Build history of the part. All positions in model axes, mm. A direction names the side the tool comes from. Round coordinates to 2 decimals unless told otherwise and drop trailing zeros. Write each loop counter-clockwise with the first axis right and the second up, starting at its lowest first coordinate (ties: lowest second). Pieces come first, ordered by that corner, then holes.
1) Saw through at A-A (z = 0). Write the cut outline in (x, y).
2) Which spindle directions (+Z, -Z, +X, -X, +Y, -Y) get a long thin tool onto all of the face, cutting with end or side? Do faces 1 (the flat face through (155, -4, 0)), 2 (the flat face through (155, 0, 5)). Say none if no direction does.
3) Saw through at C-C (y = 0). State how many separate pieces and enclosed holes the cut face has, plus the area to 3 significant figures.
4) Pull direction Z, two halves, no side cores. Call faces 3 (the flat face through (155, 4, 0)), 4 (the flat face through (155, 5, 0)), 5 (the flat face through (155, 0, -5)): +Z half, -Z half, draft (parallel to the pull), parting line (faces both ways), or undercut.
5) Saw through at B-B (x = 222). Write the cut outline in (y, z), plus the area to 3 significant figures.
6) Wall check: probe 1 along Z at (x, y) = (51.5, 1.25); probe 2 along Y at (x, z) = (307.5, -4.3). Give the ranges that are in metal, low to high.
from build123d import *

# Parameters (mm, degrees)
SKETCH_1_W          = 10
SKETCH_1_H          = 10
SKETCH_1_W_2        = 8
SKETCH_1_H_2        = 8
EXTRUDE_1_DEPTH     = 315
SKETCH_2_R          = 2.15
CUT_EXTRUDE_1_DEPTH = 316.198350249


with BuildPart() as part:
    # Sketch 1 → Extrude 1 (new body)
    with BuildSketch(Plane(origin=(0, 0, 0), x_dir=(0, 0, -1), z_dir=(1, 0, 0))):
        Rectangle(SKETCH_1_W, SKETCH_1_H)
        Rectangle(SKETCH_1_W_2, SKETCH_1_H_2, mode=Mode.SUBTRACT)
    extrude(amount=EXTRUDE_1_DEPTH)

    # Sketch 2 → Cut-Extrude 1 (cut, through all)
    with BuildSketch(Plane.XY.offset(5)):
        with Locations((307.5, 0)):
            Circle(SKETCH_2_R)
        with Locations((282.5, 0)):
            Circle(SKETCH_2_R)
        with Locations(Location((7.5, 0, 0), (0, 0, 90))):
            Circle(SKETCH_2_R)
        with Locations(Location((32.5, 0, 0), (0, 0, 90))):
            Circle(SKETCH_2_R)
        with Locations((172.5, 0)):
            Circle(SKETCH_2_R)
        with Locations((157.5, 0)):
            Circle(SKETCH_2_R)
        with Locations(Location((142.5, 0, 0), (0, 0, 90))):
            Circle(SKETCH_2_R)
    extrude(amount=-CUT_EXTRUDE_1_DEPTH, mode=Mode.SUBTRACT)


solid = part.part
Evaluation:
1. outline: (0, -5) - (315, -5) - (315, -4) - (0, -4) - close; (0, 4) - (315, 4) - (315, 5) - (0, 5) - close
2. face 1: +X, -X
2. face 2: +Z, +X, -X, +Y, -Y
3. separate pieces: 16
3. enclosed holes: 0
3. area: 570 mm2
4. face 3: undercut
4. face 4: draft
4. face 5: -Z half
5. outline: (-5, -5) - (5, -5) - (5, 5) - (-5, 5) - close; hole (-4, -4) - (4, -4) - (4, 4) - (-4, 4) - close
5. area: 36.0 mm2
6. probe 1: z = -5 to -4, 4 to 5
6. probe 2: y = -5 to -2.15, 2.15 to 5
